Autodesk Inventor part; units mm, degrees
ref_plane "YZ Plane" through (0, 0, 0) normal (1, 0, 0) x (0, 1, 0)
ref_plane "XZ Plane" through (0, 0, 0) normal (0, 1, 0) x (-1, 0, 0)
ref_plane "XY Plane" through (0, 0, 0) normal (0, 0, 1) x (1, 0, 0)
sketch "Sketch1" plane through (0, 0, 0) normal (0, 1, 0) x (-1, 0, 0)
  line L0 (0, 0) -> (441.3397, 0) construction
  line L1 (441.3397, 0) -> (441.3397, -197.552) construction
  line L2 (441.3397, -197.552) -> (0, -197.552) construction
  line L3 (0, -197.552) -> (0, 0) construction
  line L4 (171.126, -125.5766) -> (171.126, -117.3504)
  line L5 (171.126, -117.3504) -> (164.413, -117.3504)
  line L6 (164.413, -117.3504) -> (164.413, -115.3958)
  line L7 (164.413, -115.3958) -> (162.5492, -115.3958)
  line L8 (162.5492, -115.3958) -> (162.5492, -109.1021)
  line L9 (162.5492, -109.1021) -> (153.1492, -109.1021)
  line L10 (153.1492, -109.1021) -> (153.1492, -118.4751)
  line L11 (153.1492, -118.4751) -> (159.1458, -118.4751)
  line L12 (159.1458, -118.4751) -> (159.1458, -120.6901)
  line L13 (159.1458, -120.6901) -> (160.7124, -120.6901)
  line L14 (160.7124, -120.6901) -> (160.7124, -125.2266)
  line L15 (160.7124, -125.2266) -> (153.1492, -125.2266)
  line L16 (153.1492, -125.2266) -> (153.1492, -133.9258)
  line L17 (153.1492, -133.9258) -> (145.278, -133.9258)
  line L18 (145.278, -133.9258) -> (145.278, -117.3504)
  line L19 (145.278, -117.3504) -> (135.8674, -117.3504)
  line L20 (135.8674, -117.3504) -> (135.8674, -151.5449)
  line L21 (135.8674, -151.5449) -> (144.3246, -151.5449)
  line L22 (144.3246, -151.5449) -> (144.3246, -160.0944)
  line L23 (144.3246, -160.0944) -> (152.8126, -160.0944)
  line L24 (152.8126, -160.0944) -> (152.8126, -165.4456)
  line L25 (152.8126, -165.4456) -> (150.4138, -165.4456)
  line L26 (150.4138, -165.4456) -> (150.4138, -167.7828)
  line L27 (150.4138, -167.7828) -> (144.3246, -167.7828)
  line L28 (144.3246, -167.7828) -> (144.3246, -177.0397)
  line L29 (144.3246, -177.0397) -> (153.766, -177.0397)
  line L30 (153.766, -177.0397) -> (153.766, -170.9505)
  line L31 (153.766, -170.9505) -> (155.5804, -170.9505)
  line L32 (155.5804, -170.9505) -> (155.5804, -168.5671)
  line L33 (155.5804, -168.5671) -> (162.4692, -168.5671)
  line L34 (162.4692, -168.5671) -> (162.4692, -160.0944)
  line L35 (162.4692, -135.3817) -> (169.4041, -135.3817)
  line L36 (169.4041, -135.3817) -> (169.4041, -142.3165)
  line L37 (169.4041, -142.3165) -> (162.4692, -142.3165)
  line L38 (162.4692, -142.3165) -> (162.4692, -135.3817)
  line L39 (162.4692, -160.0944) -> (182.7899, -160.0944)
  line L40 (171.126, -125.5766) -> (182.7899, -125.5766)
  line L41 (194.4538, -125.5766) -> (194.4538, -117.3504)
  line L42 (194.4538, -117.3504) -> (201.1668, -117.3504)
  line L43 (201.1668, -117.3504) -> (201.1668, -115.3958)
  line L44 (201.1668, -115.3958) -> (203.0306, -115.3958)
  line L45 (203.0306, -115.3958) -> (203.0306, -109.1021)
  line L46 (203.0306, -109.1021) -> (212.4307, -109.1021)
  line L47 (212.4307, -109.1021) -> (212.4307, -118.4751)
  line L48 (212.4307, -118.4751) -> (206.4341, -118.4751)
  line L49 (206.4341, -118.4751) -> (206.4341, -120.6901)
  line L50 (206.4341, -120.6901) -> (204.8674, -120.6901)
  line L51 (204.8674, -120.6901) -> (204.8674, -125.2266)
  line L52 (204.8674, -125.2266) -> (212.4307, -125.2266)
  line L53 (212.4307, -125.2266) -> (212.4307, -133.9258)
  line L54 (212.4307, -133.9258) -> (220.3018, -133.9258)
  line L55 (220.3018, -133.9258) -> (220.3018, -117.3504)
  line L56 (220.3018, -117.3504) -> (229.7124, -117.3504)
  line L57 (229.7124, -117.3504) -> (229.7124, -151.5449)
  line L58 (229.7124, -151.5449) -> (221.2552, -151.5449)
  line L59 (221.2552, -151.5449) -> (221.2552, -160.0944)
  line L60 (221.2552, -160.0944) -> (212.7672, -160.0944)
  line L61 (212.7672, -160.0944) -> (212.7672, -165.4456)
  line L62 (212.7672, -165.4456) -> (215.166, -165.4456)
  line L63 (215.166, -165.4456) -> (215.166, -167.7828)
  line L64 (215.166, -167.7828) -> (221.2552, -167.7828)
  line L65 (221.2552, -167.7828) -> (221.2552, -177.0397)
  line L66 (221.2552, -177.0397) -> (211.8138, -177.0397)
  line L67 (211.8138, -177.0397) -> (211.8138, -170.9505)
  line L68 (211.8138, -170.9505) -> (209.9994, -170.9505)
  line L69 (209.9994, -170.9505) -> (209.9994, -168.5671)
  line L70 (209.9994, -168.5671) -> (203.1106, -168.5671)
  line L71 (203.1106, -168.5671) -> (203.1106, -160.0944)
  line L72 (203.1106, -135.3817) -> (196.1757, -135.3817)
  line L73 (196.1757, -135.3817) -> (196.1757, -142.3165)
  line L74 (196.1757, -142.3165) -> (203.1106, -142.3165)
  line L75 (203.1106, -142.3165) -> (203.1106, -135.3817)
  line L76 (203.1106, -160.0944) -> (182.7899, -160.0944)
  line L77 (194.4538, -125.5766) -> (182.7899, -125.5766)
  dimension "d17" = 90
  dimension "d18" = 6.9349
  dimension "d21" = 6.9349
  dimension "d22" = 26.6019
extrude "Extrusion1" add sketch "Sketch1" along normal blind 6.35
equation "\"d21\" = d18"
properties part number "Monster3"
Verification items for the finished model (mm, model axes). A direction names the side the tool comes from. Coordinates: 2 decimals unless noted, no trailing zeros. Order: outer loops, then holes, each group sorted by start corner. A loop starts at its lowest first (then second) coordinate and runs counter-clockwise, first axis right, second up.
1. Scan lines: line 1 (X direction, y = 0.75, z = -122); line 2 (X direction, y = 5.75, z = -136.5); line 3 (X direction, y = 4, z = -166.5). Record each from-to range of solid material in increasing order.
Results found:
line 1: x = -229.71 to -220.3, -204.87 to -194.45, -171.13 to -160.71, -145.28 to -135.87
line 2: x = -229.71 to -203.11, -196.18 to -169.4, -162.47 to -135.87
line 3: x = -215.17 to -203.11, -162.47 to -150.41
2. Sectioned sample at C-C, the plane y = 5. Give the number of separate pieces and of enclosed holes in the cut face, and give its area (3 significant figures).
Results found:
separate pieces: 1
enclosed holes: 2
area: 3,740 mm2
3. Sectioned sample at A-A, the plane z = -141. Record the cut outline in (x, y).
Results found:
outline: (-229.71, 0) - (-203.11, 0) - (-203.11, 6.35) - (-229.71, 6.35) - close; (-196.18, 0) - (-169.4, 0) - (-169.4, 6.35) - (-196.18, 6.35) - close; (-162.47, 0) - (-135.87, 0) - (-135.87, 6.35) - (-162.47, 6.35) - close
4. Go/stop test with flat-tipped pins: pin 1 Ø1.7 at (x, y) = (-159.5, 1.5) entering from -Z; pin 2 Ø3 at (x, y) = (-146.5, 3) entering from +Z; pin 3 Ø1.9 at (x, y) = (-185, 2.5) entering from +Z. Record where each tip stops, or that it passes through.
Results found:
pin 1: stops at z = -168.57
pin 2: stops at z = -117.35
pin 3: stops at z = -125.58
5. Set-up check for faces 4 (the face through (-226, 3, -151.545)), 5 (the face through (-203.031, 3, -112)), 6 (the face through (-203.111, 3, -139)), 7 (the face through (-159, 3, -168.567)): record each of +Z, -Z, +X, -X, +Y, -Y from which the full face is reachable in a straight line by a thin tool's end or side.
Results found:
face 4: -Z, -X, +Y, -Y
face 5: +Z, +Y, -Y
face 6: +Y, -Y
face 7: -Z, +Y, -Y
6. Sectioned sample at D-D, the plane x = -193. Record the cut outline in (y, z).
Results found:
outline: (0, -160.09) - (6.35, -160.09) - (6.35, -125.58) - (0, -125.58) - close
7. Sectioned sample at B-B, the plane z = -123.5. Record the cut outline in (x, y).
Results found:
outline: (-229.71, 0) - (-220.3, 0) - (-220.3, 6.35) - (-229.71, 6.35) - close; (-204.87, 0) - (-194.45, 0) - (-194.45, 6.35) - (-204.87, 6.35) - close; (-171.13, 0) - (-160.71, 0) - (-160.71, 6.35) - (-171.13, 6.35) - close; (-145.28, 0) - (-135.87, 0) - (-135.87, 6.35) - (-145.28, 6.35) - close
8. Release check for a two-part mould opening along X. For faces 1 (the face through (-212.767, 3, -163)), 2 (the face through (-147, 3, -167.783)), 3 (the face through (-169.404, 3, -139)) record: +X half, -X half, draft (parallel to the pull), parting line (faces both ways), or undercut.
Results found:
face 1: -X half
face 2: draft
face 3: undercut
